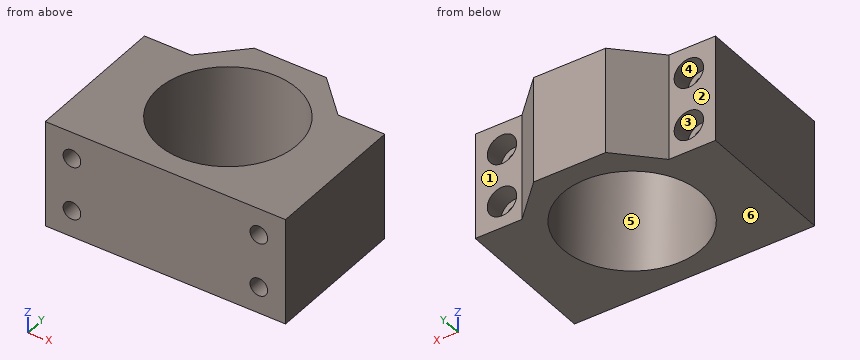
from build123d import *

# Parameters (mm, degrees)
SKETCH1_R         = 26
EXTRUSION1_DEPTH  = 40
HOLE1_D           = 6.6
HOLE1_CBORE_D     = 11
HOLE1_CBORE_DEPTH = 7.499997


with BuildPart() as part:
    # Sketch1 → Extrusion1 (new body)
    with BuildSketch(Plane.XY):
        Polygon((21.365726522, 9.909240265), (3.865726522, 9.909240265), (3.865726522, -44.090759735), (93.865726522, -44.090759735), (93.865726522, 9.909240265), (76.365726522, 9.909240265), (62.365726522, 23.909240265), (35.365726522, 23.909240265), align=None)
        with Locations((48.865726522, -10.090759735)):
            Circle(SKETCH1_R, mode=Mode.SUBTRACT)
    extrude(amount=EXTRUSION1_DEPTH)

    # Hole1 (through all)
    with Locations(Plane(origin=(0, 9.909240265, 0), x_dir=(1, 0, 0), z_dir=(0, 1, 0))):
        with Locations((13.865726522, -10), (13.865726522, -30), (83.865726522, -10), (83.865726522, -30)):
            CounterBoreHole(HOLE1_D / 2, HOLE1_CBORE_D / 2, HOLE1_CBORE_DEPTH)


solid = part.part
The model under review builds one solid part; all positions refer to its coordinate system, in mm. Face numbers are marked on the shaded views. A direction names the side the tool comes from. Round coordinates to 2 decimals unless told otherwise and drop trailing zeros. Order: outer loops, then holes, each group sorted by start corner. A loop starts at its lowest first (then second) coordinate and runs counter-clockwise, first axis right, second up. Notation, with made-up numbers: (3, 38.25) -> (46, 38.25) arc R19 cw to (46, 58.25) -> close; hole circle Ø9 at (72, 5.25). An arc over 180 degrees is marked (long way). Return JSON: item names as keys, results as strings.
1. Take a section at A-A (y = -20.5). Write out the cut boundary in (x, z), then the cut area to 3 significant figures.
Answer block:
{"outline": "(3.87, 0) -> (25.04, 0) -> (25.04, 40) -> (3.87, 40) -> close; (72.69, 0) -> (93.87, 0) -> (93.87, 40) -> (72.69, 40) -> close; hole circle Ø6.6 at (13.87, 10); hole circle Ø6.6 at (13.87, 30); hole circle Ø6.6 at (83.87, 10); hole circle Ø6.6 at (83.87, 30)", "area": "1,560 mm²"}
2. Take a section at D-D (y = 0). Write out the cut boundary in (x, z).
Answer block:
{"outline": "(3.87, 0) -> (24.9, 0) -> (24.9, 40) -> (3.87, 40) -> close; (72.83, 0) -> (93.87, 0) -> (93.87, 40) -> (72.83, 40) -> close; hole circle Ø6.6 at (13.87, 10); hole circle Ø6.6 at (13.87, 30); hole circle Ø6.6 at (83.87, 10); hole circle Ø6.6 at (83.87, 30)"}
3. Take a section at C-C (x = 25.5). Write out the cut boundary in (y, z).
Answer block:
{"outline": "(-44.09, 0) -> (-21.49, 0) -> (-21.49, 40) -> (-44.09, 40) -> close; (1.31, 0) -> (14.04, 0) -> (14.04, 40) -> (1.31, 40) -> close"}
4. For L1, parallel to X at y = -21.5, z = 30; L2, parallel to X at y = 7.5, z = 12; L3, parallel to Y at x = 18, z = 26.5, list the stretches that pass through material, from the lowest coordinate up. Write a range as [from, to].
Answer block:
{"L1": "x = [3.87, 10.57], [17.17, 25.5], [72.23, 80.57], [87.17, 93.87]", "L2": "x = [3.87, 8.74], [18.99, 29.72], [68.01, 78.74], [88.99, 93.87]", "L3": "y = [-44.09, 2.41]"}
5. Take a section at B-B (z = 10). Write out the cut boundary in (x, y), then the cut area to 3 significant figures.
Answer block:
{"outline": "(3.87, -44.09) -> (10.57, -44.09) -> (10.57, 2.41) -> (8.37, 2.41) -> (8.37, 9.91) -> (3.87, 9.91) -> close; (17.17, -44.09) -> (80.57, -44.09) -> (80.57, 2.41) -> (78.37, 2.41) -> (78.37, 9.91) -> (76.37, 9.91) -> (62.37, 23.91) -> (35.37, 23.91) -> (21.37, 9.91) -> (19.37, 9.91) -> (19.37, 2.41) -> (17.17, 2.41) -> close; (87.17, -44.09) -> (93.87, -44.09) -> (93.87, 9.91) -> (89.37, 9.91) -> (89.37, 2.41) -> (87.17, 2.41) -> close; hole circle Ø52 at (48.87, -10.09)", "area": "2,530 mm²"}
6. Insertion check: P1, Ø4, axis at x = 13.87, z = 10, coming from the -Y side; P2, Ø8, axis at x = 20.5, z = 7.5, coming from the +Y side; P3, Ø10, axis at x = 83.87, z = 30, coming from the +Y side; P4, Ø19, axis at x = 81.5, z = 17.5, coming from the +Y side. Each pin has a flat end and moves straight along its axis. Give the tip position at first contact, or say it passes through.
Answer block:
{"P1": "passes through", "P2": "stops at y = 13.04", "P3": "stops at y = 2.41", "P4": "stops at y = 14.27"}
7. For the marked faces 1, 2 and 3, list the 3-axis set-ups (+Z, -Z, +X, -X, +Y, -Y) from which the entire face can be reached by the end or side of a thin tool; tool diameter is ignored.
Answer block:
{"face 1": "+Z, -Z, +X, +Y", "face 2": "+Z, -Z, -X, +Y", "face 3": "+Y"}
8. The part is to be moulded in two halves that separate along Z. For the marked faces 4, 5 and 6, say which applies: +Z half, -Z half, draft (parallel to the pull), parting line (faces both ways), or undercut.
Answer block:
{"face 4": "undercut", "face 5": "draft", "face 6": "-Z half"}
